```python
from build123d import *

# Parameters (mm, degrees)
SKETCH1_W           = 355.6
SKETCH1_H           = 355.6
BOSS_EXTRUDE1_DEPTH = 4.826
SKETCH3_R           = 3.2639
CUT_EXTRUDE2_DEPTH  = 5.826
SKETCH5_R           = 3.2639
CUT_EXTRUDE3_DEPTH  = 5.826
SKETCH6_R           = 3.2639
CUT_EXTRUDE4_DEPTH  = 5.826


with BuildPart() as part:
    # Sketch1 → Boss-Extrude1 (new body)
    with BuildSketch(Plane(origin=(0, 0, 0), x_dir=(1, 0, 0), z_dir=(0, 1, 0))):
        Rectangle(SKETCH1_W, SKETCH1_H)
    extrude(amount=BOSS_EXTRUDE1_DEPTH)

    # Sketch3 → Cut-Extrude2 (cut, through all)
    with BuildSketch(Plane.XZ):
        with Locations((92.71, -66.04)):
            Circle(SKETCH3_R)
        with Locations((92.71, 66.04)):
            Circle(SKETCH3_R)
        with Locations((38.1, 0)):
            Circle(SKETCH3_R)
        with Locations((-38.1, 0)):
            Circle(SKETCH3_R)
        with Locations((-92.71, 66.04)):
            Circle(SKETCH3_R)
        with Locations((-92.71, -66.04)):
            Circle(SKETCH3_R)
    extrude(amount=-CUT_EXTRUDE2_DEPTH, mode=Mode.SUBTRACT)

    # Sketch5 → Cut-Extrude3 (cut, through all)
    with BuildSketch(Plane.XZ):
        with Locations((145.034, -145.034)):
            Circle(SKETCH5_R)
        with Locations((87.034, -145.034)):
            Circle(SKETCH5_R)
        with Locations((29.034, -145.034)):
            Circle(SKETCH5_R)
        with Locations((-28.966, -145.034)):
            Circle(SKETCH5_R)
        with Locations((-86.966, -145.034)):
            Circle(SKETCH5_R)
        with Locations((-144.966, -145.034)):
            Circle(SKETCH5_R)
        with Locations((145.034, -87.034)):
            Circle(SKETCH5_R)
        with Locations((87.034, -87.034)):
            Circle(SKETCH5_R)
        with Locations((29.034, -87.034)):
            Circle(SKETCH5_R)
        with Locations((-28.966, -87.034)):
            Circle(SKETCH5_R)
        with Locations((-86.966, -87.034)):
            Circle(SKETCH5_R)
        with Locations((-144.966, -87.034)):
            Circle(SKETCH5_R)
        with Locations((145.034, -29.034)):
            Circle(SKETCH5_R)
        with Locations((87.034, -29.034)):
            Circle(SKETCH5_R)
        with Locations((29.034, -29.034)):
            Circle(SKETCH5_R)
        with Locations((-28.966, -29.034)):
            Circle(SKETCH5_R)
        with Locations((-86.966, -29.034)):
            Circle(SKETCH5_R)
        with Locations((-144.966, -29.034)):
            Circle(SKETCH5_R)
        with Locations((145.034, 28.966)):
            Circle(SKETCH5_R)
        with Locations((87.034, 28.966)):
            Circle(SKETCH5_R)
        with Locations((29.034, 28.966)):
            Circle(SKETCH5_R)
        with Locations((-28.966, 28.966)):
            Circle(SKETCH5_R)
        with Locations((-86.966, 28.966)):
            Circle(SKETCH5_R)
        with Locations((-144.966, 28.966)):
            Circle(SKETCH5_R)
        with Locations((145.034, 86.966)):
            Circle(SKETCH5_R)
        with Locations((87.034, 86.966)):
            Circle(SKETCH5_R)
        with Locations((29.034, 86.966)):
            Circle(SKETCH5_R)
        with Locations((-28.966, 86.966)):
            Circle(SKETCH5_R)
        with Locations((-86.966, 86.966)):
            Circle(SKETCH5_R)
        with Locations((-144.966, 86.966)):
            Circle(SKETCH5_R)
        with Locations((145.034, 144.966)):
            Circle(SKETCH5_R)
        with Locations((87.034, 144.966)):
            Circle(SKETCH5_R)
        with Locations((29.034, 144.966)):
            Circle(SKETCH5_R)
        with Locations((-28.966, 144.966)):
            Circle(SKETCH5_R)
        with Locations((-86.966, 144.966)):
            Circle(SKETCH5_R)
        with Locations((-144.966, 144.966)):
            Circle(SKETCH5_R)
    extrude(amount=-CUT_EXTRUDE3_DEPTH, mode=Mode.SUBTRACT)

    # Sketch6 → Cut-Extrude4 (cut, through all)
    with BuildSketch(Plane.XZ):
        with Locations((116.034, -116.034)):
            Circle(SKETCH6_R)
        with Locations((58.034, -116.034)):
            Circle(SKETCH6_R)
        with Locations((0.034, -116.034)):
            Circle(SKETCH6_R)
        with Locations((-57.966, -116.034)):
            Circle(SKETCH6_R)
        with Locations((-115.966, -116.034)):
            Circle(SKETCH6_R)
        with Locations((116.034, -58.034)):
            Circle(SKETCH6_R)
        with Locations((58.034, -58.034)):
            Circle(SKETCH6_R)
        with Locations((0.034, -58.034)):
            Circle(SKETCH6_R)
        with Locations((-57.966, -58.034)):
            Circle(SKETCH6_R)
        with Locations((-115.966, -58.034)):
            Circle(SKETCH6_R)
        with Locations((116.034, -0.034)):
            Circle(SKETCH6_R)
        with Locations((58.034, -0.034)):
            Circle(SKETCH6_R)
        with Locations((0.034, -0.034)):
            Circle(SKETCH6_R)
        with Locations((-57.966, -0.034)):
            Circle(SKETCH6_R)
        with Locations((-115.966, -0.034)):
            Circle(SKETCH6_R)
        with Locations((116.034, 57.966)):
            Circle(SKETCH6_R)
        with Locations((58.034, 57.966)):
            Circle(SKETCH6_R)
        with Locations((0.034, 57.966)):
            Circle(SKETCH6_R)
        with Locations((-57.966, 57.966)):
            Circle(SKETCH6_R)
        with Locations((-115.966, 57.966)):
            Circle(SKETCH6_R)
        with Locations((116.034, 115.966)):
            Circle(SKETCH6_R)
        with Locations((58.034, 115.966)):
            Circle(SKETCH6_R)
        with Locations((0.034, 115.966)):
            Circle(SKETCH6_R)
        with Locations((-57.966, 115.966)):
            Circle(SKETCH6_R)
        with Locations((-115.966, 115.966)):
            Circle(SKETCH6_R)
    extrude(amount=-CUT_EXTRUDE4_DEPTH, mode=Mode.SUBTRACT)


solid = part.part
```
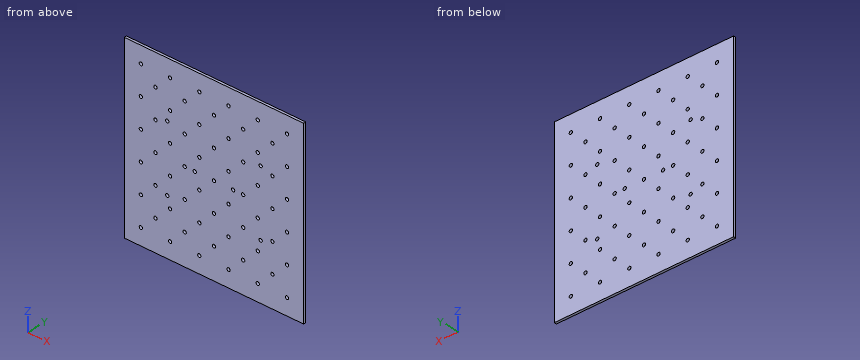
Model file for the job. Use its own axes, mm. Coordinates: 2 decimals unless noted, no trailing zeros. Answer as a JSON object with one key per item and string values. Group by question number.
1) Flat gauge pins, fed straight in: pin 1 (6 mm diameter, centred on x = -115.966, z = 115.966, fed in from -Y); pin 2 (7.5 mm diameter, centred on x = 145.034, z = 86.966, fed in from +Y). Where does each tip first touch, or does it go through?
2) Drill centre lines: L1, parallel to X at y = 2.2, z = 65.5; L2, parallel to Z at x = -94.5, y = 1.8; L3, parallel to X at y = 1.6, z = -57. Where is each one in solid material? Low to high.
3) Cut at A-A, the plane y = 4. Count the separate pieces of the cut face and the enclosed holes in it, then the cut area to 3 significant figures.
Check values:
{
 "1": {"pin 1": "passes through", "pin 2": "stops at y = 4.83"},
 "2": {"L1": "x = -177.8 to -95.93, -89.49 to 89.49, 95.93 to 177.8", "L2": "z = -177.8 to -68.77, -63.31 to 63.31, 68.77 to 177.8", "L3": "x = -177.8 to -119.06, -112.87 to -61.06, -54.87 to -3.06, 3.13 to 54.94, 61.13 to 112.94, 119.13 to 177.8"},
 "3": {"separate pieces": "1", "enclosed holes": "67", "area": "124,000 mm²"}
}
